Part print with two shaded views. Sizes in mm from the minimum x, y, z corner. A direction names the side the tool comes from. Round coordinates to 2 decimals unless told otherwise and drop trailing zeros. Order: outer loops, then holes, each group sorted by start corner. A loop starts at its lowest first (then second) coordinate and runs counter-clockwise, first axis right, second up. Notation, with made-up numbers: M 27,29 L 42,29 A21 ccw 42,65 Z; hole C -26,78.25 d8. An arc over 180 degrees is marked long. Answer as a JSON object with one key per item and string values.
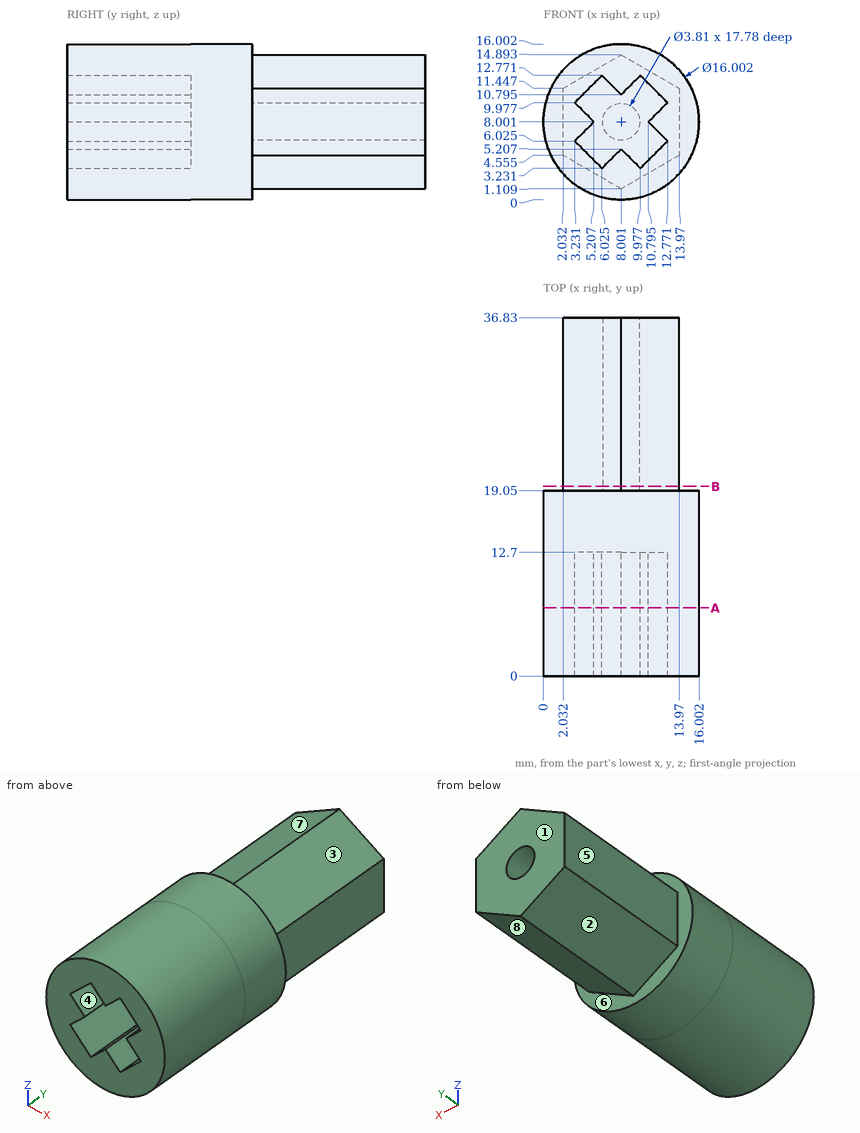
Item 1: Saw through at A-A on y = 7. List the corners of the cut face in (x, z) (1 decimal).
Worked answers:
{"outline": "C 8,8 d16; hole M 3.2,6 L 6,3.2 L 8,5.2 L 10,3.2 L 12.8,6 L 10.8,8 L 12.8,10 L 10,12.8 L 8,10.8 L 6,12.8 L 3.2,10 L 5.2,8 Z"}
Item 2: Wall check: line 1 along Z through (x, y) = (11.25, 9.5) (1 decimal); line 2 along X through (y, z) = (10, 11) (1 decimal); line 3 along Y through (x, z) = (3.5, 14.25). Give the ranges that are in metal, low to high. Write a range as [from, to].
Worked answers:
{"line 1": "z = [0.7, 4.5], [7.5, 8.5], [11.5, 15.3]", "line 2": "x = [0.6, 4.3], [7.8, 8.2], [11.7, 15.4]", "line 3": "y = [0, 19.05]"}
Item 3: Drop flat-ended pins along their axis: pin 1 Ø3 at (y, z) = (15, 7) entering from -X; pin 2 Ø7.5 at (y, z) = (32, 8.5) entering from -X; pin 3 Ø1.5 at (x, y) = (12.5, 8.5) entering from +Z; pin 4 Ø1.9 at (x, z) = (8, 7.5) entering from +Y. Give the stop position or say it passes through.
Worked answers:
{"pin 1": "stops at x = 0", "pin 2": "stops at x = 2.03", "pin 3": "stops at z = 15.07", "pin 4": "stops at y = 19.05"}
Item 4: Two-plate mould, pull along X, no slides. Class the marked faces 1, 2, 3 and 4: released by +X, released by -X, zero draft, split by the parting line, or undercut.
Worked answers:
{"face 1": "zero draft", "face 2": "released by -X", "face 3": "released by +X", "face 4": "undercut"}
Item 5: Saw through at B-B on y = 19.5. List the corners of the cut face in (x, z) (1 decimal), and give its area (3 significant figures).
Worked answers:
{"outline": "M 2,4.6 L 8,1.1 L 14,4.6 L 14,11.4 L 8,14.9 L 2,11.4 Z; hole C 8,8 d3.8", "area": "112 mm2"}
Item 6: 3-axis set-ups, long thin cutter, end or side, ignore diameter. For the marked faces 5, 6, 7 and 8: which of +Z, -Z, +X, -X, +Y, -Y reach the whole face in a straight line?
Worked answers:
{"face 5": "+Z, -Z, -X, +Y", "face 6": "+Y", "face 7": "+Z, -X, +Y", "face 8": "-Z, +X, +Y"}
